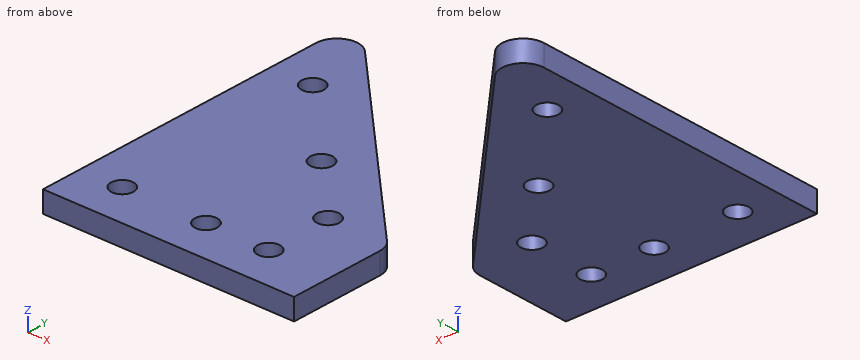
```python
from build123d import *

# Parameters (mm, degrees)
BOSS_EXTRUDE1_DEPTH     = 3.175
F_1_4_CLEARANCE_HOLE1_D = 6.7564
FILLET1_R               = 6.35


with BuildPart() as part:
    # Sketch1 → Boss-Extrude1 (new, symmetric)
    with BuildSketch(Plane.XY):
        Polygon((-38.1, -15.875), (38.1, -15.875), (38.1, 15.875), (-38.1, 92.075), align=None)
    extrude(amount=BOSS_EXTRUDE1_DEPTH, both=True)

    # 1/4 Clearance Hole1 (through all)
    with Locations(Plane.XY.offset(3.175)):
        with Locations((-25.4, 61.414487758), (0, 36.014487758), (19.05, 16.964487758), (-25.4, -3.175), (19.05, -3.175), (0, -3.175)):
            Hole(F_1_4_CLEARANCE_HOLE1_D / 2)

    # Fillet1
    fillet1_edges = [part.edges().sort_by_distance(p)[0] for p in [
        (-38.1, 92.075, 0),
        (38.1, 15.875, 0),
    ]]
    fillet(fillet1_edges, radius=FILLET1_R)


solid = part.part
```
The listing builds one solid part. Answer for the finished solid, in the listing's coordinates (mm). Give positions to 0.01 mm unless a question says otherwise; leave off trailing zeros. Order: outer loops, then holes, each group sorted by start corner. A loop starts at its lowest first (then second) coordinate and runs counter-clockwise, first axis right, second up. Notation, with made-up numbers: (-29, -28.5) - (-6, -28.5) arc R24 ccw to (-6, -3.5) - close; hole circle Ø7 at (78, -11.5). An arc over 180 degrees is marked (long way). Answer in a Markdown table with one row per item. Add a question column.
Q1. The part is cut by section B-B (z = -0.5). Determine the outline of the cut face in (x, y) (3 decimals), then the cut area to 3 significant figures.
Q2. The part is cut by section D-D (y = 42). Determine the outline of the cut face in (x, z) (3 decimals).
Q3. Find the intervals of material crossed by line 1 along X through (y, z) = (-4, -1); line 2 along Y through (x, z) = (-25.4, 1.25) (3 decimals); line 3 along X through (y, z) = (-6, 1.5), in increasing order. Write a range as [from, to].
Q4. The part is cut by section A-A (x = 19.05). Determine the outline of the cut face in (y, z) (3 decimals).
Q5. The part is cut by section C-C (x = -25.4). Determine the outline of the cut face in (y, z) (3 decimals), then the cut area to 3 significant figures.
Determined:
| question | item | result |
|---|---|---|
| 1 | outline | (-38.1, -15.875) - (38.1, -15.875) - (38.1, 13.245) arc R6.35 ccw to (36.24, 17.735) - (-27.26, 81.235) arc R6.35 ccw to (-38.1, 76.745) - close; hole circle Ø6.756 at (-25.4, -3.175); hole circle Ø6.756 at (-25.4, 61.414); hole circle Ø6.756 at (0, -3.175); hole circle Ø6.756 at (0, 36.014); hole circle Ø6.756 at (19.05, -3.175); hole circle Ø6.756 at (19.05, 16.964) |
| 1 | area | 5,060 mm² |
| 2 | outline | (-38.1, -3.175) - (11.975, -3.175) - (11.975, 3.175) - (-38.1, 3.175) - close |
| 3 | line 1 | x = [-38.1, -28.68], [-22.12, -3.28], [3.28, 15.77], [22.33, 38.1] |
| 3 | line 2 | y = [-15.875, -6.553], [0.203, 58.036], [64.793, 79.375] |
| 3 | line 3 | x = [-38.1, -27.25], [-23.55, -1.85], [1.85, 17.2], [20.9, 38.1] |
| 4 | outline | (-15.875, -3.175) - (-6.553, -3.175) - (-6.553, 3.175) - (-15.875, 3.175) - close; (0.203, -3.175) - (13.586, -3.175) - (13.586, 3.175) - (0.203, 3.175) - close; (20.343, -3.175) - (34.925, -3.175) - (34.925, 3.175) - (20.343, 3.175) - close |
| 5 | outline | (-15.875, -3.175) - (-6.553, -3.175) - (-6.553, 3.175) - (-15.875, 3.175) - close; (0.203, -3.175) - (58.036, -3.175) - (58.036, 3.175) - (0.203, 3.175) - close; (64.793, -3.175) - (79.375, -3.175) - (79.375, 3.175) - (64.793, 3.175) - close |
| 5 | area | 519 mm² |
